from build123d import *

# Parameters (mm, degrees)
SKETCH_1_W          = 70
SKETCH_1_H          = 100
EXTRUDE_1_DEPTH     = 3
SKETCH_2_R          = 2
CUT_EXTRUDE_1_DEPTH = 123.102416029
SKETCH_3_W          = 9.819716148
SKETCH_3_H          = 21.548821549
SKETCH_3_W_2        = 11.047180667
SKETCH_3_H_2        = 24.549290372
SKETCH_3_W_3        = 2.454929037
SKETCH_3_H_3        = 3.273238716
SKETCH_3_W_4        = 1.909389251
SKETCH_3_W_5        = 2.318544091
SKETCH_3_W_6        = 4.364318288
SKETCH_3_H_4        = 2.045774198
SKETCH_3_H_5        = 2.182159144
SKETCH_3_H_6        = 2.591313983
EXTRUDE_2_DEPTH     = 3
SKETCH_4_W          = 6.582292946
SKETCH_4_H          = 14.208853527
SKETCH_4_W_2        = 20.616767863
SKETCH_4_H_2        = 5.990006879
EXTRUDE_3_DEPTH     = 6


with BuildPart() as part:
    # Эскиз1 → Бобышка-Вытянуть1 (new body)
    with BuildSketch(Plane.XY):
        with Locations((35, 50)):
            Rectangle(SKETCH_1_W, SKETCH_1_H)
    extrude(amount=EXTRUDE_1_DEPTH)

    # Эскиз2 → Вырез-Вытянуть1 (cut, through all)
    with BuildSketch(Plane.XY.offset(3)):
        with Locations((8, 92)):
            Circle(SKETCH_2_R)
        with Locations((62, 92)):
            Circle(SKETCH_2_R)
        with Locations(Location((62, 8, 0), (0, 0, 180))):
            Circle(SKETCH_2_R)
        with Locations(Location((8, 8, 0), (0, 0, 180))):
            Circle(SKETCH_2_R)
    extrude(amount=-CUT_EXTRUDE_1_DEPTH, mode=Mode.SUBTRACT)

    # Эскиз3 → Бобышка-Вытянуть2 (add)
    with BuildSketch(Plane.XY.offset(3)):
        with Locations((28.589907514, 64.252226911)):
            Rectangle(SKETCH_3_W, SKETCH_3_H)
        with Locations((48.161147339, 30.292375229)):
            Rectangle(SKETCH_3_W_2, SKETCH_3_H_2)
        with Locations((12.632868773, 35.065848357)):
            Rectangle(SKETCH_3_W_3, SKETCH_3_H_3)
        with Locations((20.679580617, 35.065848357)):
            Rectangle(SKETCH_3_W_4, SKETCH_3_H_3)
        with Locations((27.430635469, 35.065848357)):
            Rectangle(SKETCH_3_W_5, SKETCH_3_H_3)
        with Locations((51.502578528, 67.866427993)):
            Rectangle(SKETCH_3_W_6, SKETCH_3_H_4)
        with Locations((51.502578528, 73.935558113)):
            Rectangle(SKETCH_3_W_6, SKETCH_3_H_5)
        with Locations((51.502578528, 79.186378554)):
            Rectangle(SKETCH_3_W_6, SKETCH_3_H_6)
    extrude(amount=EXTRUDE_2_DEPTH)

    # Эскиз4 → Бобышка-Вытянуть3 (add)
    with BuildSketch(Plane.XY.offset(3)):
        with Locations((3.291146473, 66.880429277)):
            Rectangle(SKETCH_4_W, SKETCH_4_H)
        with Locations((28.313480694, 12.343506182)):
            Rectangle(SKETCH_4_W_2, SKETCH_4_H_2)
    extrude(amount=EXTRUDE_3_DEPTH)


solid = part.part
The model under review builds one solid part; all positions refer to its coordinate system, in mm. A direction names the side the tool comes from. Round coordinates to 2 decimals unless told otherwise and drop trailing zeros. Loops run counter-clockwise (first coordinate to the right, second up) from the corner with the lowest first, then second, coordinate; pieces in that order, holes last. Notation, with made-up numbers: M 49.25,87.5 L 99.25,87.5 A16 ccw 99.25,93.5 Z; hole C 19.25,-27 d6. An arc over 180 degrees is marked long. Answer as CSV lines item,"result". Start each with the question number.
Item 1: Consider section B-B (z = 7.75). Write out the cut boundary in (x, y).
Item 2: Wall thickness on line 1 (Y direction, x = 8, z = 1.9); line 2 (X direction, y = 35, z = 4); line 3 (Y direction, x = 32.5, z = 5.5): over which ranges is each line inside the solid? List them lowest first. Write a range as [from, to].
Item 3: Insertion check: P1, Ø1.5, axis at x = 51.5, z = 4.5, coming from the +Y side; P2, Ø3, axis at x = 21, z = 6.5, coming from the -Y side; P3, Ø3.5, axis at y = 67.5, z = 4.5, coming from the -X side; P4, Ø1.6, axis at x = 52.5, y = 68, coming from the +Z side. Each pin has a flat end and moves straight along its axis. Give the tip position at first contact, or say it passes through.
Item 4: Consider section D-D (y = 61). Write out the cut boundary in (x, z).
Item 5: Consider section C-C (x = 8). Write out the cut boundary in (y, z), then the cut area to 3 significant figures.
Item 6: Consider section A-A (y = 92). Write out the cut boundary in (x, z).
Item 7: For faces 1 (the face through (49.32, 68, 4)), 2 (the face through (51, 80.482, 4)), 3 (the face through (26.271, 35, 4)), 4 (the face through (51, 75.027, 4)), list the 3-axis set-ups (+Z, -Z, +X, -X, +Y, -Y) from which the entire face can be reached by the end or side of a thin tool; tool diameter is ignored.
Item 8: Mouldability with a two-part tool opening along Y and no side actions: class faces 5 (the face through (11.405, 35, 4)), 6 (the face through (62, 94, 2)), 7 (the face through (35, 100, 1)) as released by +Y, released by -Y, zero draft, split by the parting line, or undercut.
Answer:
1,outline,"M 0,59.78 L 6.58,59.78 L 6.58,73.98 L 0,73.98 Z; M 18.01,9.35 L 38.62,9.35 L 38.62,15.34 L 18.01,15.34 Z"
2,line 1,"y = [0, 6], [10, 90], [94, 100]"
2,line 2,"x = [11.41, 13.86], [19.72, 21.63], [26.27, 28.59], [42.64, 53.68]"
2,line 3,"y = [9.35, 15.34], [53.48, 75.03]"
3,P1,"stops at y = 80.48"
3,P2,"stops at y = 9.35"
3,P3,"stops at x = 0"
3,P4,"stops at z = 6"
4,outline,"M 0,0 L 70,0 L 70,3 L 33.5,3 L 33.5,6 L 23.68,6 L 23.68,3 L 6.58,3 L 6.58,9 L 0,9 Z"
5,outline,"M 0,0 L 6,0 L 6,3 L 0,3 Z; M 10,0 L 90,0 L 90,3 L 10,3 Z; M 94,0 L 100,0 L 100,3 L 94,3 Z"
5,area,"276 mm^2"
6,outline,"M 0,0 L 6,0 L 6,3 L 0,3 Z; M 10,0 L 60,0 L 60,3 L 10,3 Z; M 64,0 L 70,0 L 70,3 L 64,3 Z"
7,face 1,"+Z, +Y"
7,face 2,"+Z, +X, -X, +Y"
7,face 3,"+Z"
7,face 4,"+Z, +X, -X"
8,face 5,"zero draft"
8,face 6,"undercut"
8,face 7,"released by +Y"
